from build123d import *

# Parameters (mm, degrees)
PAD002_DEPTH           = 30
POCKET_DEPTH           = 4.5
LINEARPATTERN_COUNT    = 2
LINEARPATTERN_PITCH    = 16
SKETCH003_R            = 2.25
HOLE_DEPTH             = 25
LINEARPATTERN001_COUNT = 2
LINEARPATTERN001_PITCH = 16


with BuildPart() as part:
    # Sketch002 → Pad002 (new body)
    with BuildSketch(Plane.XY):
        Polygon((0, 0), (0, 8), (-4, 8), (-7.9, 4.1), (-7.9, 2.2), (-3.75, 2.2), (-3.75, 0), align=None)
    pad002 = extrude(amount=PAD002_DEPTH)

    # Mirrored: Pad002 across Sketch002 V_Axis
    add(pad002.mirror(Plane(origin=(0, 0, 0), x_dir=(0, 0, 1), z_dir=(1, 0, 0))))

    # Sketch (on DatumPlane) → Pocket (cut)
    with BuildSketch(Plane(origin=(0, 8, 0), x_dir=(-1, 0, 0), z_dir=(0, 1, 0))):
        Polygon((0, 2.727608), (3.7, 4.863804), (3.7, 9.136196), (0, 11.272392), (-3.7, 9.136196), (-3.7, 4.863804), align=None)
    pocket = extrude(amount=-POCKET_DEPTH, mode=Mode.SUBTRACT)

    # LinearPattern: Pocket ×2
    with Locations(*[(0, 0, i * LINEARPATTERN_PITCH) for i in range(1, LINEARPATTERN_COUNT)]):
        add(pocket, mode=Mode.SUBTRACT)

    # Sketch003 (on DatumPlane) → Hole (cut)
    with BuildSketch(Plane(origin=(0, 8, 0), x_dir=(-1, 0, 0), z_dir=(0, 1, 0))):
        with Locations((0, 7.3)):
            Circle(SKETCH003_R)
    hole = extrude(amount=-HOLE_DEPTH, mode=Mode.SUBTRACT)

    # LinearPattern001: Hole ×2
    with Locations(*[(0, 0, i * LINEARPATTERN001_PITCH) for i in range(1, LINEARPATTERN001_COUNT)]):
        add(hole, mode=Mode.SUBTRACT)


solid = part.part
Part model, mm, in its own coordinate system. A direction names the side the tool comes from. Round coordinates to 2 decimals unless told otherwise and drop trailing zeros. Order: outer loops, then holes, each group sorted by start corner. A loop starts at its lowest first (then second) coordinate and runs counter-clockwise, first axis right, second up. Notation, with made-up numbers: (4.5, 32.25) -> (52.5, 32.25) arc R19 cw to (52.5, 68.25) -> close; hole circle Ø11 at (66.5, -15). An arc over 180 degrees is marked (long way). Put each result on its own line as item: value.
Q1. Tool access for faces 1 (the face through (3.75, 1, 15)), 2 (the face through (-7.9, 3, 15)), 3 (the face through (3.7, 6, 7)): list every direction of +Z, -Z, +X, -X, +Y, -Y with a clear straight run to the whole face (end or side of a thin tool).
From the geometry:
face 1: +Z, -Z, +X, -Y
face 2: +Z, -Z, -X, +Y, -Y
face 3: +Y
Q2. Band-saw the part on A-A (z = 23.3). Give the cut face in (x, y), and give its area (3 significant figures).
From the geometry:
outline: (-7.9, 2.2) -> (-3.75, 2.2) -> (-3.75, 0) -> (-2.25, 0) -> (-2.25, 3.5) -> (-3.7, 3.5) -> (-3.7, 8) -> (-4, 8) -> (-7.9, 4.1) -> close; (2.25, 0) -> (3.75, 0) -> (3.75, 2.2) -> (7.9, 2.2) -> (7.9, 4.1) -> (4, 8) -> (3.7, 8) -> (3.7, 3.5) -> (2.25, 3.5) -> close
area: 43.9 mm2
Q3. Band-saw the part on D-D (z = 20.25). Give the cut face in (x, y).
From the geometry:
outline: (-7.9, 2.2) -> (-3.75, 2.2) -> (-3.75, 0) -> (3.75, 0) -> (3.75, 2.2) -> (7.9, 2.2) -> (7.9, 4.1) -> (4, 8) -> (2.64, 8) -> (2.64, 3.5) -> (-2.64, 3.5) -> (-2.64, 8) -> (-4, 8) -> (-7.9, 4.1) -> close
Q4. Pull direction Z, two halves, no side cores. Call faces 4 (the face through (1, 3.5, 5)), 5 (the face through (6, 6, 15)), 6 (the face through (0, 4, 0)), 7 (the face through (0, 4, 30)): pulls with the +Z half, pulls with the -Z half, needs draft (parallel to the pull), parting line crosses it, or undercut.
From the geometry:
face 4: undercut
face 5: needs draft
face 6: pulls with the -Z half
face 7: pulls with the +Z half
Q5. Band-saw the part on C-C (y = 0.5). Give the cut face in (x, z), and give its area (3 significant figures).
From the geometry:
outline: (-3.75, 0) -> (3.75, 0) -> (3.75, 30) -> (-3.75, 30) -> close; hole circle Ø4.5 at (0, 7.3); hole circle Ø4.5 at (0, 23.3)
area: 193 mm2
Q6. Band-saw the part on B-B (x = -1.25). Give the cut face in (y, z).
From the geometry:
outline: (0, 0) -> (8, 0) -> (8, 3.45) -> (3.5, 3.45) -> (3.5, 5.43) -> (0, 5.43) -> close; (0, 9.17) -> (3.5, 9.17) -> (3.5, 10.55) -> (8, 10.55) -> (8, 19.45) -> (3.5, 19.45) -> (3.5, 21.43) -> (0, 21.43) -> close; (0, 25.17) -> (3.5, 25.17) -> (3.5, 26.55) -> (8, 26.55) -> (8, 30) -> (0, 30) -> close
Q7. Wall check: line 1 (Z direction, x = 0, y = 1.6); line 2 (Z direction, x = 0.75, y = 6.25); line 3 (X direction, y = 3.25, z = 9.25). Give the ranges that are in metal, low to high. Write a range as [from, to].
From the geometry:
line 1: z = [0, 5.05], [9.55, 21.05], [25.55, 30]
line 2: z = [0, 3.16], [10.84, 19.16], [26.84, 30]
line 3: x = [-7.9, -1.12], [1.12, 7.9]
Q8. Pin check, flat tips, straight feed: pin 1 Ø1.3 at (y, z) = (5, 22.5) entering from +X; pin 2 Ø3.5 at (x, z) = (0, 7.3) entering from -Y; pin 3 Ø3.5 at (x, z) = (1, 24) entering from +Y; pin 4 Ø2 at (y, z) = (6, 22) entering from -X. Stop position of each tip, or through.
From the geometry:
pin 1: stops at x = 7.65
pin 2: passes through
pin 3: stops at y = 3.5
pin 4: stops at x = -7
